The listing builds one solid part. Answer for the finished solid, in the listing's coordinates (mm). Face numbers are marked on the shaded views. A direction names the side the tool comes from. Round coordinates to 2 decimals unless told otherwise and drop trailing zeros. Order: outer loops, then holes, each group sorted by start corner. A loop starts at its lowest first (then second) coordinate and runs counter-clockwise, first axis right, second up. Notation, with made-up numbers: (47, -21) - (58, -21) arc R31 cw to (58, 3) - close; hole circle Ø4 at (51.25, 66). An arc over 180 degrees is marked (long way). One line per item, written item: value. Start each with the question number.
1. Section A-A, the plane z = 6.5 is taken. Give the vertices of the cut face in (x, y), then the cut area to 3 significant figures.
2. A tool of negligible diameter and unlimited length cuts with its end or side. For the marked faces 1, 2 and 3, from which of +Z, -Z, +X, -X, +Y, -Y can it reach the whole face along a straight path? Write none if from no direction.
3. Flat-ended cylindrical pins translate along their axes: P1, Ø5.5, axis at x = -33.5, y = 33.5, coming from the -Z side; P2, Ø1.2, axis at x = 0, y = -44.5, coming from the +Z side; P3, Ø1.7, axis at y = -36, z = -27, coming from the -X side. Find the tip coordinate at first contact, or state that the pin passes through.
4. Section D-D, the plane z = -19 is taken. Give the vertices of the cut face in (x, y), then the cut area to 3 significant figures.
5. For a pull along X with two mould halves and no side action, classify the marked faces 4, 5, 6 and 7 as released by +X, released by -X, zero draft, split by the parting line, or undercut.
6. Straight lines are drawn through the part: line 1 (Y direction, x = 0, z = 8); line 2 (Y direction, x = 0, z = -68); line 3 (Y direction, x = 23, z = -48.5). For each, find the intervals that lie inside material, in ascending order.
7. Section B-B, the plane y = 0 is taken. Give the vertices of the cut face in (x, z), then the cut area to 3 significant figures.
from build123d import *

# Parameters (mm, degrees)
SKETCH_1_W                  = 86
SKETCH_1_H                  = 86
EXTRUDE_1_DEPTH             = 78.1
SKETCH_2_R                  = 36.5
EXTRUDE_2_DEPTH             = 1.5
HOLE_WIZARD_M30_1_D         = 35
HOLE_WIZARD_M30_1_DEPTH     = 6.5
SKETCH_5_R                  = 6.35
EXTRUDE_3_DEPTH             = 36.75
CUT_EXTRUDE_START           = -25
CUT_EXTRUDE_1_DEPTH         = 25
SKETCH_7_W                  = 69.6
SKETCH_7_H                  = 13.95
CUT_EXTRUDE_2_DEPTH         = 13.95
SKETCH_8_W                  = 13.95
SKETCH_8_H                  = 69.6
CUT_EXTRUDE_3_DEPTH         = 13.95
SKETCH_9_W                  = 13.95
SKETCH_9_H                  = 13.95
CUT_EXTRUDE_4_DEPTH         = 69.6
SKETCH_10_W                 = 13.95
SKETCH_10_H                 = 13.95
CUT_EXTRUDE_5_DEPTH         = 69.6
EXTRUDE_4_DEPTH             = 2.5
SKETCH_12_R                 = 3
EXTRUDE_5_DEPTH             = 27.5
HOLE_WIZARD_6_5_6_5_1_D     = 6.5
HOLE_WIZARD_6_5_6_5_1_DEPTH = 78.1
HOLE_WIZARD_6_5_6_5_2_D     = 6.5
HOLE_WIZARD_6_5_6_5_2_DEPTH = 40.25
HOLE_WIZARD_M27_1_D         = 32
HOLE_WIZARD_M27_1_DEPTH     = 4.4
FILLET_1_R                  = 4.6
FILLET_2_R                  = 5.5
FILLET_3_R                  = 5.9


with BuildPart() as part:
    # 草图1 → 凸台-拉伸1 (new body)
    with BuildSketch(Plane(origin=(0, 0, -69.6), x_dir=(-1, 0, 0), z_dir=(0, 0, -1))):
        Rectangle(SKETCH_1_W, SKETCH_1_H)
    extrude(amount=-EXTRUDE_1_DEPTH)

    # 草图2 → 凸台-拉伸2 (add)
    with BuildSketch(Plane.XY.offset(8.5)):
        with Locations(Location((0, 0, 0), (0, 0, 180))):
            Circle(SKETCH_2_R)
    extrude(amount=EXTRUDE_2_DEPTH)

    # M30 间隙孔1
    with Locations(Plane.XY.offset(10)):
        with Locations((0, 0)):
            Hole(HOLE_WIZARD_M30_1_D / 2, depth=HOLE_WIZARD_M30_1_DEPTH)

    # 草图5 → 凸台-拉伸3 (add)
    with BuildSketch(Plane.XY.offset(3.5)):
        with Locations(Location((0, 0, 0), (0, 0, 180))):
            Circle(SKETCH_5_R)
    extrude(amount=EXTRUDE_3_DEPTH)

    # 草图6 → 切除-拉伸1 (cut)
    with BuildSketch(Plane.XY.offset(40.25).offset(CUT_EXTRUDE_START)):
        with BuildLine():
            Line((-3.527619594, 5.28), (3.527619595, 5.28))
            ThreePointArc((3.527619595, 5.28), (1e-09, 6.35), (-3.527619594, 5.28))
        make_face()
    extrude(amount=CUT_EXTRUDE_1_DEPTH, mode=Mode.SUBTRACT)

    # 草图7 → 切除-拉伸2 (cut)
    with BuildSketch(Plane.ZY.offset(43)):
        with Locations((-34.8, 36.025)):
            Rectangle(SKETCH_7_W, SKETCH_7_H)
    extrude(amount=-CUT_EXTRUDE_2_DEPTH, mode=Mode.SUBTRACT)

    # 草图8 → 切除-拉伸3 (cut)
    with BuildSketch(Plane(origin=(0, 43, 0), x_dir=(-1, 0, 0), z_dir=(0, 1, 0))):
        with Locations((-36.025, -34.8)):
            Rectangle(SKETCH_8_W, SKETCH_8_H)
    extrude(amount=-CUT_EXTRUDE_3_DEPTH, mode=Mode.SUBTRACT)

    # 草图9 → 切除-拉伸4 (cut)
    with BuildSketch(Plane(origin=(0, 0, -69.6), x_dir=(-1, 0, 0), z_dir=(0, 0, -1))):
        with Locations((36.025, -36.025)):
            Rectangle(SKETCH_9_W, SKETCH_9_H)
    extrude(amount=-CUT_EXTRUDE_4_DEPTH, mode=Mode.SUBTRACT)

    # 草图10 → 切除-拉伸5 (cut)
    with BuildSketch(Plane(origin=(0, 0, -69.6), x_dir=(-1, 0, 0), z_dir=(0, 0, -1))):
        with Locations((-36.025, -36.025)):
            Rectangle(SKETCH_10_W, SKETCH_10_H)
    extrude(amount=-CUT_EXTRUDE_5_DEPTH, mode=Mode.SUBTRACT)

    # 草图11 → 凸台-拉伸4 (add)
    with BuildSketch(Plane.XZ.offset(43)):
        with BuildLine():
            Line((-5, -56.987641526), (5, -56.987641526))
            Line((5, -56.987641526), (5, -63.287641526))
            ThreePointArc((5, -63.287641526), (0, -68.287641526), (-5, -63.287641526))
            Line((-5, -63.287641526), (-5, -56.987641526))
        make_face()
    extrude(amount=EXTRUDE_4_DEPTH)

    # 草图12 → 凸台-拉伸5 (add)
    with BuildSketch(Plane.XZ.offset(45.5)):
        with Locations(Location((0, -63.287641526, 0), (0, 0, 90))):
            Circle(SKETCH_12_R)
    extrude(amount=EXTRUDE_5_DEPTH)

    # Ø6.5 (6.5) 直径孔1
    with Locations(Plane.XY.offset(8.5)):
        with Locations((34.789653634, -34.789653634)):
            Hole(HOLE_WIZARD_6_5_6_5_1_D / 2, depth=HOLE_WIZARD_6_5_6_5_1_DEPTH)

    # Ø6.5 (6.5) 直径孔2
    with Locations(Plane(origin=(0, 0, 0), x_dir=(-1, 0, 0), z_dir=(0, 0, -1))):
        with Locations((34.789653634, -34.789653634), (-34.789653634, 34.789653634), (34.789653634, 34.789653634)):
            Hole(HOLE_WIZARD_6_5_6_5_2_D / 2, depth=HOLE_WIZARD_6_5_6_5_2_DEPTH)

    # M27 间隙孔1
    with Locations(Plane(origin=(0, 0, -69.6), x_dir=(-1, 0, 0), z_dir=(0, 0, -1))):
        with Locations((0, 0)):
            Hole(HOLE_WIZARD_M27_1_D / 2, depth=HOLE_WIZARD_M27_1_DEPTH)

    # 圆角1
    fillet_1_edges = [part.edges().sort_by_distance(p)[0] for p in [
        (-29.05, 43, -34.8),
        (-43, 29.05, -34.8),
        (43, 29.05, -34.8),
        (29.05, 43, -34.8),
        (-43, -29.05, -34.8),
        (-29.05, -43, -34.8),
        (29.05, -43, -34.8),
        (43, -29.05, -34.8),
    ]]
    fillet(fillet_1_edges, radius=FILLET_1_R)

    # 圆角2
    fillet_2_edges = [part.edges().sort_by_distance(p)[0] for p in [
        (-43, -43, 4.25),
        (43, -43, 4.25),
        (43, 43, 4.25),
        (-43, 43, 4.25),
    ]]
    fillet(fillet_2_edges, radius=FILLET_2_R)

    # 圆角3
    fillet_3_edges = [part.edges().sort_by_distance(p)[0] for p in [
        (-29.05, 29.05, -34.8),
        (29.05, 29.05, -34.8),
        (-29.05, -29.05, -34.8),
        (29.05, -29.05, -34.8),
    ]]
    fillet(fillet_3_edges, radius=FILLET_3_R)


solid = part.part
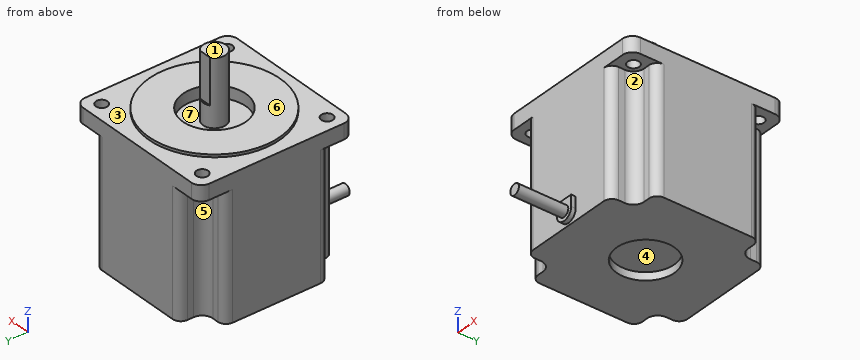
Answer list:
1. outline: (-43, -37.5) arc R5.5 ccw to (-37.5, -43) - (37.5, -43) arc R5.5 ccw to (43, -37.5) - (43, 37.5) arc R5.5 ccw to (37.5, 43) - (-37.5, 43) arc R5.5 ccw to (-43, 37.5) - close; circle Ø12.7 at (0, 0); hole circle Ø6.5 at (-34.79, -34.79); hole circle Ø6.5 at (-34.79, 34.79); hole circle Ø35 at (0, 0); hole circle Ø6.5 at (34.79, -34.79); hole circle Ø6.5 at (34.79, 34.79)
1. area: 6,400 mm²
2. face 1: +Z, +X, -X, +Y, -Y
2. face 2: -Z, +X, -Y
2. face 3: +Z
3. P1: stops at z = 0
3. P2: stops at z = -56.99
3. P3: stops at x = -29.05
4. outline: (-43, -24.45) arc R4.6 ccw to (-38.4, -29.05) - (-34.95, -29.05) arc R5.9 cw to (-29.05, -34.95) - (-29.05, -38.4) arc R4.6 ccw to (-24.45, -43) - (24.45, -43) arc R4.6 ccw to (29.05, -38.4) - (29.05, -34.95) arc R5.9 cw to (34.95, -29.05) - (38.4, -29.05) arc R4.6 ccw to (43, -24.45) - (43, 24.45) arc R4.6 ccw to (38.4, 29.05) - (34.95, 29.05) arc R5.9 cw to (29.05, 34.95) - (29.05, 38.4) arc R4.6 ccw to (24.45, 43) - (-24.45, 43) arc R4.6 ccw to (-29.05, 38.4) - (-29.05, 34.95) arc R5.9 cw to (-34.95, 29.05) - (-38.4, 29.05) arc R4.6 ccw to (-43, 24.45) - close
4. area: 6,610 mm²
5. face 4: undercut
5. face 5: released by -X
5. face 6: zero draft
5. face 7: undercut
6. line 1: y = -43 to -17.5, -6.35 to 6.35, 17.5 to 43
6. line 2: y = -45.5 to -16, 16 to 43
6. line 3: y = -43 to 43
7. outline: (-43, -69.6) - (-16, -69.6) - (-16, -65.2) - (16, -65.2) - (16, -69.6) - (43, -69.6) - (43, 8.5) - (36.5, 8.5) - (36.5, 10) - (17.5, 10) - (17.5, 3.5) - (6.35, 3.5) - (6.35, 40.25) - (-6.35, 40.25) - (-6.35, 3.5) - (-17.5, 3.5) - (-17.5, 10) - (-36.5, 10) - (-36.5, 8.5) - (-43, 8.5) - close
7. area: 6,920 mm²
